from build123d import *

# Parameters (mm, degrees)
SKETCH1_R           = 34
SKETCH1_R_2         = 1.6999999999999995
SKETCH1_R_3         = 1.7
SKETCH1_R_4         = 13
BOSS_EXTRUDE1_DEPTH = 2
SKETCH3_R           = 40.37992907465996
CUT_EXTRUDE1_DEPTH  = 2
SKETCH4_R           = 5.000000000000001
SKETCH4_R_2         = 1.6999999999999995
BOSS_EXTRUDE2_DEPTH = 1
CIRPATTERN1_COUNT   = 3
FILLET1_ANGLE       = 68.695952
FILLET1_2_ANGLE     = 68.695952
FILLET1_3_ANGLE     = 68.695952


with BuildPart() as part:
    # Sketch1 → Boss-Extrude1 (new body)
    with BuildSketch(Plane(origin=(0, 0, 0), x_dir=(1, 0, 0), z_dir=(0, 1, 0))):
        with Locations(Location((0, 0, 0), (0, 0, 270))):
            Circle(SKETCH1_R)
        with Locations(Location((15.58845, 8.99999580374902, 0), (0, 0, 270))):
            Circle(SKETCH1_R_2, mode=Mode.SUBTRACT)
        with Locations(Location((1.73e-15, -17.999991607498043, 0), (0, 0, 270))):
            Circle(SKETCH1_R_3, mode=Mode.SUBTRACT)
        with Locations(Location((-15.588449999999993, 8.999995803749012, 0), (0, 0, 270))):
            Circle(SKETCH1_R_2, mode=Mode.SUBTRACT)
        with Locations(Location((0, 0, 0), (0, 0, 270))):
            Circle(SKETCH1_R_4, mode=Mode.SUBTRACT)
    extrude(amount=BOSS_EXTRUDE1_DEPTH)

    # Sketch3 → Cut-Extrude1 (cut)
    with BuildSketch(Plane(origin=(0, 2, 0), x_dir=(1, 0, 0), z_dir=(0, 1, 0))):
        with Locations((51.96152422706632, -29.999999999999986)):
            Circle(SKETCH3_R)
    cut_extrude1 = extrude(amount=-CUT_EXTRUDE1_DEPTH, mode=Mode.SUBTRACT)

    # Sketch4 → Boss-Extrude2 (add)
    with BuildSketch(Plane(origin=(0, 2, 0), x_dir=(1, 0, 0), z_dir=(0, 1, 0))):
        with Locations(Location((-15.588449999999993, 8.999995803749012, 0), (0, 0, 330))):
            Circle(SKETCH4_R)
        with Locations(Location((-15.588449999999993, 8.999995803749012, 0), (0, 0, 270))):
            Circle(SKETCH4_R_2, mode=Mode.SUBTRACT)
    boss_extrude2 = extrude(amount=BOSS_EXTRUDE2_DEPTH)

    # CirPattern1: Cut-Extrude1, Boss-Extrude2 ×3 about axis
    cirpattern1_axis = Axis((-1.58e-15, 0, 2.4e-16), (0, 1, 0))
    add([cut_extrude1.rotate(cirpattern1_axis, i * 360 / CIRPATTERN1_COUNT) for i in range(1, CIRPATTERN1_COUNT)], mode=Mode.SUBTRACT)
    add([boss_extrude2.rotate(cirpattern1_axis, i * 360 / CIRPATTERN1_COUNT) for i in range(1, CIRPATTERN1_COUNT)])

    # Fillet1: read off the stored shape, not the designer's step
    # Fillet1 outline → Fillet1 (revolve, cut)
    with BuildSketch(Plane(origin=(0, 0, -60), x_dir=(-0.5642175786181923, 0, 0.8256261405613463), z_dir=(-0.8256261405613463, 0, -0.5642175786181923))):
        with BuildLine():
            ThreePointArc((40.379929075, 0), (43.217651415, 1.486832981), (46.379929075, 2))
            Line((46.379929075, 2), (40.379929075, 2))
            Line((40.379929075, 2), (40.379929075, 0))
        make_face()
    revolve(axis=Axis((0, 0, -60), (0, 1, 0)), revolution_arc=FILLET1_ANGLE, mode=Mode.SUBTRACT)

    # Fillet1 2 outline → Fillet1 2 (revolve, cut)
    with BuildSketch(Plane(origin=(-51.961524227, 0, 30), x_dir=(0.9971220010637243, 0, 0.07581368606441925), z_dir=(-0.07581368606441925, 0, 0.9971220010637243))):
        with BuildLine():
            ThreePointArc((40.379929075, 0), (43.217651415, 1.486832981), (46.379929075, 2))
            Line((46.379929075, 2), (40.379929075, 2))
            Line((40.379929075, 2), (40.379929075, 0))
        make_face()
    revolve(axis=Axis((-51.961524227, 0, 30), (0, 1.0000000000000002, 0)), revolution_arc=FILLET1_2_ANGLE, mode=Mode.SUBTRACT)

    # Fillet1 3 outline → Fillet1 3 (revolve, cut)
    with BuildSketch(Plane(origin=(51.961524227, 0, 30), x_dir=(-0.43290442244553945, 0, -0.9014398266257676), z_dir=(0.9014398266257676, 0, -0.43290442244553945))):
        with BuildLine():
            ThreePointArc((40.379929075, 0), (43.217651415, 1.486832981), (46.379929075, 2))
            Line((46.379929075, 2), (40.379929075, 2))
            Line((40.379929075, 2), (40.379929075, 0))
        make_face()
    revolve(axis=Axis((51.961524227, 0, 30), (0, 1, 0)), revolution_arc=FILLET1_3_ANGLE, mode=Mode.SUBTRACT)


solid = part.part
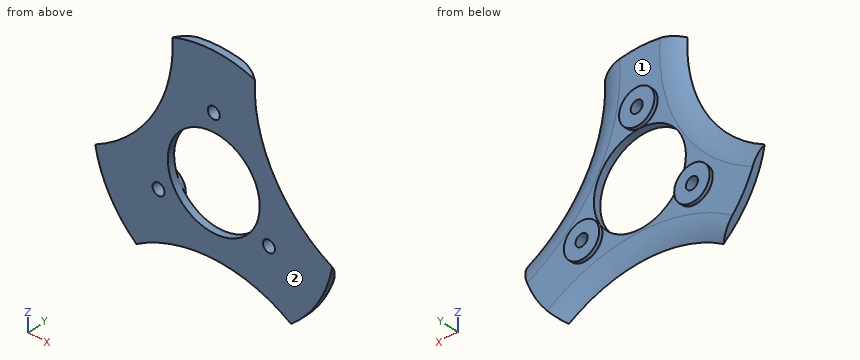
Can you work these out from the model? Positions are in its coordinate system, mm. Face numbers are marked on the shaded views. A direction names the side the tool comes from. Round coordinates to 2 decimals unless told otherwise and drop trailing zeros. Order: outer loops, then holes, each group sorted by start corner. A loop starts at its lowest first (then second) coordinate and runs counter-clockwise, first axis right, second up. Notation, with made-up numbers: (43, 47) - (47, 47) arc R6 cw to (47, 56) - close; hole circle Ø4 at (80, -0.5). An arc over 180 degrees is marked (long way). Answer in a Markdown table with one row per item.
(1) Suppose I cut it at A-A, the plane y = 1.4. Please give me the cut outline in (x, z).
From the geometry:
| item | result |
|---|---|
| outline | (-32.92, -8.52) arc R34 ccw to (-23.83, -24.25) arc R42.97 cw to (23.83, -24.25) arc R34 ccw to (32.92, -8.52) arc R42.97 cw to (9.08, 32.76) arc R34 ccw to (-9.08, 32.76) arc R42.97 cw to start; hole circle Ø3.4 at (-15.59, -9); hole circle Ø26 at (0, 0); hole circle Ø3.4 at (0, 18); hole circle Ø3.4 at (15.59, -9) |
(2) Which directions (+Z, -Z, +X, -X, +Y, -Y) give clear straight access to the entire face, cutting with the end or side of a thin tool? Please do the marked faces 1 and 2.
From the geometry:
| item | result |
|---|---|
| face 1 | +Y |
| face 2 | +Z, -Z, +X, -X, -Y |
(3) Please list where these lines run through material, in increasing order: L1, parallel to Z at x = 1.5, y = 0.95; L2, parallel to X at y = 0.85, z = 8.5; L3, parallel to Y at x = -4, z = 28. Write a range as from..to.
From the geometry:
| item | result |
|---|---|
| L1 | z = -18.11..-12.91, 12.91..17.2, 18.8..33.97 |
| L2 | x = -16.2..-9.84, 9.84..16.2 |
| L3 | y = 0..2 |
(4) For P1, Ø2, axis at x = 20.5, z = -19.5, coming from the +Y side; P2, Ø1.5, axis at y = 1.5, z = 5, coming from the -X side, each with a flat end and sliding along its axis, tell me the tip position at first contact or that it passes through.
From the geometry:
| item | result |
|---|---|
| P1 | stops at y = 2 |
| P2 | stops at x = -18.88 |
